Can you work these out from the model? Positions are in its coordinate system, mm. A direction names the side the tool comes from. Round coordinates to 2 decimals unless told otherwise and drop trailing zeros. Loops run counter-clockwise (first coordinate to the right, second up) from the corner with the lowest first, then second, coordinate; pieces in that order, holes last. Notation, with made-up numbers: (-35, -1.75) -> (-29, -1.75) arc R26 cw to (-29, 37.25) -> close; hole circle Ø9 at (16, 76). An arc over 180 degrees is marked (long way). Answer as a JSON object with one key per item and string values.
```python
from build123d import *

# Parameters (mm, degrees)
SKETCH1_R                                    = 11
BOSS_EXTRUDE1_DEPTH                          = 2.5
CSK_FOR_M3_SOCKET_COUNTERSUNK_HEAD_S_2_COUNT = 2
CSK_FOR_M3_SOCKET_COUNTERSUNK_HEAD_S_2_PITCH = 10.606601718
CSK_FOR_M3_SOCKET_COUNTERSUNK_HEAD_S_3_COUNT = 2
CSK_FOR_M3_SOCKET_COUNTERSUNK_HEAD_S_3_PITCH = 15
CSK_FOR_M3_SOCKET_COUNTERSUNK_HEAD_S_4_COUNT = 2
CSK_FOR_M3_SOCKET_COUNTERSUNK_HEAD_S_4_PITCH = 10.606601718
CUT_EXTRUDE1_DEPTH                           = 16.755951257


with BuildPart() as part:
    # Sketch1 → Boss-Extrude1 (new body)
    with BuildSketch(Plane(origin=(0, 0, 0), x_dir=(1, 0, 0), z_dir=(0, 1, 0))):
        with Locations(Location((0, 0, 0), (0, 0, 270))):
            Circle(SKETCH1_R)
    extrude(amount=BOSS_EXTRUDE1_DEPTH)

    # Sketch3 → CSK for M3 socket countersunk head screw1 (revolve, cut)
    with BuildSketch(Plane(origin=(-7.5, 2.5, 0), x_dir=(0, 0, 1), z_dir=(1, 0, 0))):
        Polygon((0, 0), (0, 2.5), (1.7, 2.5), (1.7, 1.4), (3.1, 0), align=None)
    csk_for_m3_socket_countersunk_head_screw = revolve(axis=Axis((-7.5, 8.85, 0), (0, -1, 0)), mode=Mode.SUBTRACT)

    # CSK for M3 socket countersunk head s 2: CSK for M3 socket countersunk head screw1 ×2
    with Locations(*[Vector(0.7071067811865303, 0, -0.7071067811865648) * (i * CSK_FOR_M3_SOCKET_COUNTERSUNK_HEAD_S_2_PITCH) for i in range(1, CSK_FOR_M3_SOCKET_COUNTERSUNK_HEAD_S_2_COUNT)]):
        add(csk_for_m3_socket_countersunk_head_screw, mode=Mode.SUBTRACT)

    # CSK for M3 socket countersunk head s 3: CSK for M3 socket countersunk head screw1 ×2
    with Locations(*[(i * CSK_FOR_M3_SOCKET_COUNTERSUNK_HEAD_S_3_PITCH, 0, 0) for i in range(1, CSK_FOR_M3_SOCKET_COUNTERSUNK_HEAD_S_3_COUNT)]):
        add(csk_for_m3_socket_countersunk_head_screw, mode=Mode.SUBTRACT)

    # CSK for M3 socket countersunk head s 4: CSK for M3 socket countersunk head screw1 ×2
    with Locations(*[Vector(0.7071067811865648, 0, 0.7071067811865303) * (i * CSK_FOR_M3_SOCKET_COUNTERSUNK_HEAD_S_4_PITCH) for i in range(1, CSK_FOR_M3_SOCKET_COUNTERSUNK_HEAD_S_4_COUNT)]):
        add(csk_for_m3_socket_countersunk_head_screw, mode=Mode.SUBTRACT)

    # Sketch4 → Cut-Extrude1 (cut, through all)
    with BuildSketch(Plane(origin=(0, 2.5, 0), x_dir=(1, 0, 0), z_dir=(0, 1, 0))):
        with BuildLine():
            Line((-2.085965005, 3.853731957), (-3.853731957, 2.085965005))
            Line((-3.853731957, 2.085965005), (-3.00520382, 1.237436867))
            ThreePointArc((-3.00520382, 1.237436867), (2.298097039, -2.298097039), (-1.237436867, 3.00520382))
            Line((-1.237436867, 3.00520382), (-2.085965005, 3.853731957))
        make_face()
    extrude(amount=-CUT_EXTRUDE1_DEPTH, mode=Mode.SUBTRACT)


solid = part.part
```
Q1. I want a section at D-D, the plane z = -7.5. Write out the boundary of the cut face in (x, y), then the cut area to 3 significant figures.
Determined:
{"outline": "(-8.05, 0) -> (-1.7, 0) -> (-1.7, 1.1) -> (-3.1, 2.5) -> (-8.05, 2.5) -> close; (1.7, 0) -> (8.05, 0) -> (8.05, 2.5) -> (3.1, 2.5) -> (1.7, 1.1) -> close", "area": "29.8 mm²"}
Q2. I want a section at C-C, the plane y = 0.7. Write out the boundary of the cut face in (x, z), then the cut area to 3 significant figures.
Determined:
{"outline": "circle Ø22 at (0, 0); hole circle Ø3.4 at (-7.5, 0); hole (-3.85, -2.09) -> (-2.09, -3.85) -> (-1.24, -3.01) arc R3.25 ccw (long way) to (-3.01, -1.24) -> close; hole circle Ø3.4 at (0, -7.5); hole circle Ø3.4 at (0, 7.5); hole circle Ø3.4 at (7.5, 0)", "area": "308 mm²"}
Q3. I want a section at B-B, the plane x = 0. Write out the boundary of the cut face in (y, z).
Determined:
{"outline": "(0, -11) -> (2.5, -11) -> (2.5, -10.6) -> (1.1, -9.2) -> (0, -9.2) -> close; (0, -5.8) -> (1.1, -5.8) -> (2.5, -4.4) -> (2.5, -3.25) -> (0, -3.25) -> close; (0, 3.25) -> (2.5, 3.25) -> (2.5, 4.4) -> (1.1, 5.8) -> (0, 5.8) -> close; (0, 9.2) -> (1.1, 9.2) -> (2.5, 10.6) -> (2.5, 11) -> (0, 11) -> close"}
Q4. We'd pull the mould along X, two halves only. Please class faces 1 (the flat face through (3, 0, 2)), 2 (the flat face through (-3.44, 1.27, -1.67)), 3 (the cylindrical face through (-10.74, 1.23, -2.38)): pulls with the +X half, pulls with the -X half, needs draft (parallel to the pull), parting line crosses it, or undercut.
Determined:
{"face 1": "needs draft", "face 2": "undercut", "face 3": "parting line crosses it"}
Q5. If I drill on L1, parallel to X at y = 0.8, z = 0; L2, parallel to X at y = 2.3, z = -0.25; L3, parallel to Z at x = -9.5, y = 2.25, over which ranges is the centre line in solid material (lowest first)? Write a range as [from, to].
Determined:
{"L1": "[-11, -9.2], [-5.8, -3.25], [3.25, 5.8], [9.2, 11]", "L2": "[-11, -10.39], [-4.61, -3.24], [3.24, 4.61], [10.39, 11]", "L3": "[-5.55, -2.03], [2.03, 5.55]"}
Q6. I want a section at A-A, the plane z = 0. Write out the boundary of the cut face in (x, y), then the cut area to 3 significant figures.
Determined:
{"outline": "(-11, 0) -> (-9.2, 0) -> (-9.2, 1.1) -> (-10.6, 2.5) -> (-11, 2.5) -> close; (-5.8, 0) -> (-3.25, 0) -> (-3.25, 2.5) -> (-4.4, 2.5) -> (-5.8, 1.1) -> close; (3.25, 0) -> (5.8, 0) -> (5.8, 1.1) -> (4.4, 2.5) -> (3.25, 2.5) -> close; (9.2, 0) -> (11, 0) -> (11, 2.5) -> (10.6, 2.5) -> (9.2, 1.1) -> close", "area": "17.8 mm²"}
Q7. I'm going to push flat-ended pins straight in: pin 1 (1.5 mm diameter, centred on y = 0.5, z = 1.5, fed in from -X); pin 2 (1 mm diameter, centred on x = 6.5, y = 1, fed in from -Z); pin 3 (2.5 mm diameter, centred on x = -7.5, z = 0, fed in from +Y). Where does each tip first touch, or does it pass through?
Determined:
{"pin 1": "x = -10.97", "pin 2": "z = -9.22", "pin 3": "through"}
Q8. On a 3-axis mill with a long thin cutter (end or side, diameter ignored), from which of +Z, -Z, +X, -X, +Y, -Y can I reach the whole of each face in a straight line? I mean faces 4 (the flat face through (3, 2.5, 2)), 5 (the flat face through (-1.656, 1.268, -3.424)). Say none if no direction works.
Determined:
{"face 4": "+Z, -Z, +X, -X, +Y", "face 5": "+Y, -Y"}
